CAD build for the part. Positions are in the model's coordinates, mm. Face numbers are marked on the shaded views. A direction names the side the tool comes from. Round coordinates to 2 decimals unless told otherwise and drop trailing zeros. Write each loop counter-clockwise with the first axis right and the second up, starting at its lowest first coordinate (ties: lowest second). Pieces come first, ordered by that corner, then holes. Notation, with made-up numbers: (13.25, -30.75) - (20.25, -30.75) arc R18 ccw to (20.25, -22.75) - close; hole circle Ø6 at (-5, -17.5). An arc over 180 degrees is marked (long way). Answer in a Markdown table with one row per item.
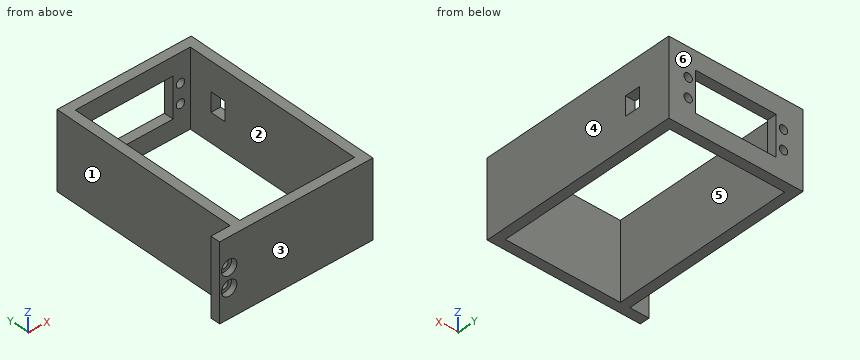
```python
from build123d import *

# Parameters (mm, degrees)
SKETCH2_W           = 80
SKETCH2_H           = 40
SKETCH2_R           = 2.2
BOSS_EXTRUDE1_DEPTH = 5
SKETCH3_W           = 5
SKETCH3_H           = 40
BOSS_EXTRUDE2_DEPTH = 100
SKETCH4_W           = 10
SKETCH4_H           = 8
CUT_EXTRUDE1_DEPTH  = 10
SKETCH5_W           = 40
SKETCH5_H           = 5
BOSS_EXTRUDE3_DEPTH = 70
SKETCH6_R           = 2.2
SKETCH6_W           = 42
SKETCH6_H           = 21
CUT_EXTRUDE2_DEPTH  = 70
SKETCH7_R           = 4
SKETCH7_R_2         = 2.2
CUT_EXTRUDE3_DEPTH  = 3


with BuildPart() as part:
    # Sketch2 → Boss-Extrude1 (new body)
    with BuildSketch(Plane(origin=(0, 0, 0), x_dir=(1, 0, 0), z_dir=(0, 1, 0))):
        with Locations((-40, 20)):
            Rectangle(SKETCH2_W, SKETCH2_H)
        with Locations((-75, 25)):
            Circle(SKETCH2_R, mode=Mode.SUBTRACT)
        with Locations((-75, 15)):
            Circle(SKETCH2_R, mode=Mode.SUBTRACT)
    extrude(amount=BOSS_EXTRUDE1_DEPTH)

    # Sketch3 → Boss-Extrude2 (add)
    with BuildSketch(Plane(origin=(0, 5, 0), x_dir=(1, 0, 0), z_dir=(0, 1, 0))):
        with Locations((-2.5, 20)):
            Rectangle(SKETCH3_W, SKETCH3_H)
        with Locations((-67.5, 20)):
            Rectangle(SKETCH3_W, SKETCH3_H)
    extrude(amount=BOSS_EXTRUDE2_DEPTH)

    # Sketch4 → Cut-Extrude1 (cut)
    with BuildSketch(Plane(origin=(0, 0, 0), x_dir=(0, 0, -1), z_dir=(1, 0, 0))):
        with Locations((20, 84)):
            Rectangle(SKETCH4_W, SKETCH4_H)
    extrude(amount=-CUT_EXTRUDE1_DEPTH, mode=Mode.SUBTRACT)

    # Sketch5 → Boss-Extrude3 (add)
    with BuildSketch(Plane(origin=(0, 0, 0), x_dir=(0, 0, -1), z_dir=(1, 0, 0))):
        with Locations((20, 102.5)):
            Rectangle(SKETCH5_W, SKETCH5_H)
    extrude(amount=-BOSS_EXTRUDE3_DEPTH)

    # Sketch6 → Cut-Extrude2 (cut)
    with BuildSketch(Plane(origin=(0, 105, 0), x_dir=(1, 0, 0), z_dir=(0, 1, 0))):
        with Locations((-59.89, 25)):
            Circle(SKETCH6_R)
        with Locations((-59.89, 15)):
            Circle(SKETCH6_R)
        with Locations((-10.11, 15)):
            Circle(SKETCH6_R)
        with Locations((-10.11, 25)):
            Circle(SKETCH6_R)
        with Locations((-35, 20)):
            Rectangle(SKETCH6_W, SKETCH6_H)
    extrude(amount=-CUT_EXTRUDE2_DEPTH, mode=Mode.SUBTRACT)

    # Sketch7 → Cut-Extrude3 (cut)
    with BuildSketch(Plane.XZ):
        with Locations((-75, -15)):
            Circle(SKETCH7_R)
        with Locations((-75, -15)):
            Circle(SKETCH7_R_2, mode=Mode.SUBTRACT)
        with Locations((-75, -25)):
            Circle(SKETCH7_R)
        with Locations((-75, -25)):
            Circle(SKETCH7_R_2, mode=Mode.SUBTRACT)
    extrude(amount=-CUT_EXTRUDE3_DEPTH, mode=Mode.SUBTRACT)


solid = part.part
```
Q1. Flat gauge pins, fed straight in: pin 1 (4 mm diameter, centred on y = 103.5, z = -23.5, fed in from -X); pin 2 (7 mm diameter, centred on x = -75, z = -25, fed in from +Y). Where does each tip first touch, or does it go through?
Computed:
| item | result |
|---|---|
| pin 1 | stops at x = -70 |
| pin 2 | stops at y = 5 |
Q2. Saw through at B-B on x = -75. List the corners of the cut face in (y, z), then the cut area to 3 significant figures.
Computed:
| item | result |
|---|---|
| outline | (0, -40) - (5, -40) - (5, -27.2) - (3, -27.2) - (3, -29) - (0, -29) - close; (0, -21) - (3, -21) - (3, -22.8) - (5, -22.8) - (5, -17.2) - (3, -17.2) - (3, -19) - (0, -19) - close; (0, -11) - (3, -11) - (3, -12.8) - (5, -12.8) - (5, 0) - (0, 0) - close |
| area | 134 mm2 |
Q3. Saw through at D-D on z = -3. List the corners of the cut face in (x, y).
Computed:
| item | result |
|---|---|
| outline | (-80, 0) - (0, 0) - (0, 105) - (-70, 105) - (-70, 5) - (-80, 5) - close; hole (-65, 5) - (-5, 5) - (-5, 100) - (-65, 100) - close |
Q4. Drill centre lines: line 1 (Z direction, x = -10.11, y = 102.25); line 2 (X direction, y = 36, z = -34); line 3 (Y direction, x = -30.5, z = -31.5). Where is each one in solid material? Low to high.
Computed:
| item | result |
|---|---|
| line 1 | z = -40 to -27.2, -22.8 to -17.2, -12.8 to 0 |
| line 2 | x = -70 to -65, -5 to 0 |
| line 3 | y = 0 to 5, 100 to 105 |
Q5. Saw through at C-C on x = -10.11. List the corners of the cut face in (y, z), then the cut area to 3 significant figures.
Computed:
| item | result |
|---|---|
| outline | (0, -40) - (5, -40) - (5, 0) - (0, 0) - close; (100, -40) - (105, -40) - (105, -27.2) - (100, -27.2) - close; (100, -22.8) - (105, -22.8) - (105, -17.2) - (100, -17.2) - close; (100, -12.8) - (105, -12.8) - (105, 0) - (100, 0) - close |
| area | 356 mm2 |
Q6. Pull direction X, two halves, no side cores. Call the marked faces 1, 2, 3 and 4: released by +X, released by -X, zero draft, split by the parting line, or undercut.
Computed:
| item | result |
|---|---|
| face 1 | released by -X |
| face 2 | undercut |
| face 3 | zero draft |
| face 4 | released by +X |
Q7. 3-axis set-ups, long thin cutter, end or side, ignore diameter. For the marked faces 5 and 6: which of +Z, -Z, +X, -X, +Y, -Y reach the whole face in a straight line?
Computed:
| item | result |
|---|---|
| face 5 | +Z, -Z |
| face 6 | +Z, -Z, +X, -X, +Y |
Q8. Saw through at A-A on y = 31.5. List the corners of the cut face in (x, z).
Computed:
| item | result |
|---|---|
| outline | (-70, -40) - (-65, -40) - (-65, 0) - (-70, 0) - close; (-5, -40) - (0, -40) - (0, 0) - (-5, 0) - close |
